Verification items for the finished model (mm, model axes). Give positions to 0.01 mm unless a question says otherwise; leave off trailing zeros. Loops run counter-clockwise (first coordinate to the right, second up) from the corner with the lowest first, then second, coordinate; pieces in that order, holes last. Notation, with made-up numbers: (84, 4.5) - (92, 4.5) arc R26 ccw to (92, 43.5) - close; hole circle Ø11 at (85, 21). An arc over 180 degrees is marked (long way). One line per question, with ' | ' between items. Start each with the question number.
1. Section check B-B, the plane y = -33.25. Enter the section's corners in (x, z).
2. Depth check by flat-ended pin: pin 1 Ø8 at (x, z) = (-51, 64.5) entering from +Y; pin 2 Ø1.5 at (x, z) = (-43, 56.5) entering from +Y. Enter the tip coordinate at first touch or a pass-through.
3. Section check C-C, the plane z = 60. Enter the section's corners in (x, y).
4. Section check A-A, the plane x = -37.5. Enter the section's corners in (y, z).
5. Thickness scan on line 1 along Y through (x, z) = (-35.5, 59); line 2 along X through (y, z) = (-47, 62.5); line 3 along Y through (x, z) = (-36, 70). Record the ranges inside material, lowest first. Write a range as from..to.
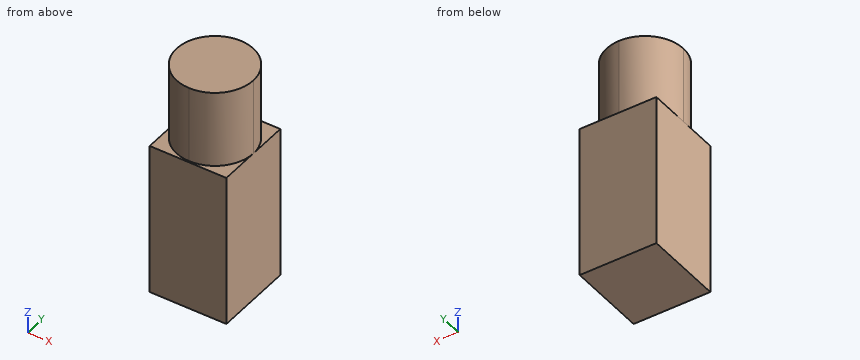
from build123d import *

# Parameters (mm, degrees)
F0_W     = 25.4
F0_H     = 26.3435523957
F1_DEPTH = 50.8
F3_DEPTH = 25.4


with BuildPart() as f1:
    # F0 (on Top) → F1 (new body)
    with BuildSketch(Plane.XY):
        with Locations((-44.2919794798, -43.9860569313)):
            Rectangle(F0_W, F0_H)
    extrude(amount=F1_DEPTH)

    # F2 (on face) → F3 (join)
    with BuildSketch(Plane.XY.offset(50.8)):
        with BuildLine():
            Line((-31.5919794798, -43.9860569313), (-44.2919794798, -43.9860569313))
            Line((-44.2919794798, -43.9860569313), (-44.2919794798, -56.6860569313))
            ThreePointArc((-44.2919794798, -56.6860569313), (-35.3117233587, -52.9663130524), (-31.5919794798, -43.9860569313))
        make_face()
        with BuildLine():
            ThreePointArc((-31.5919794798, -43.9860569313), (-35.3117233587, -35.0058008102), (-44.2919794798, -31.2860569313))
            Line((-44.2919794798, -31.2860569313), (-44.2919794798, -43.9860569313))
            Line((-44.2919794798, -43.9860569313), (-31.5919794798, -43.9860569313))
        make_face()
        with BuildLine():
            Line((-44.2919794798, -43.9860569313), (-44.2919794798, -31.2860569313))
            ThreePointArc((-44.2919794798, -31.2860569313), (-53.2722356009, -35.0058008102), (-56.9919794798, -43.9860569313))
            Line((-56.9919794798, -43.9860569313), (-44.2919794798, -43.9860569313))
        make_face()
        with BuildLine():
            Line((-44.2919794798, -56.6860569313), (-44.2919794798, -43.9860569313))
            Line((-44.2919794798, -43.9860569313), (-56.9919794798, -43.9860569313))
            ThreePointArc((-56.9919794798, -43.9860569313), (-53.2722356009, -52.9663130524), (-44.2919794798, -56.6860569313))
        make_face()
    extrude(amount=F3_DEPTH)


solid = f1.part
Results list:
1) outline: (-56.99, 0) - (-31.59, 0) - (-31.59, 50.8) - (-37.51, 50.8) - (-37.51, 76.2) - (-51.08, 76.2) - (-51.08, 50.8) - (-56.99, 50.8) - close
2) pin 1: y = -31.58 | pin 2: y = -31.3
3) outline: circle Ø25.4 at (-44.29, -43.99)
4) outline: (-57.16, 0) - (-30.81, 0) - (-30.81, 50.8) - (-33.25, 50.8) - (-33.25, 76.2) - (-54.72, 76.2) - (-54.72, 50.8) - (-57.16, 50.8) - close
5) line 1: -53.15..-34.82 | line 2: -56.63..-31.95 | line 3: -53.61..-34.37
